from build123d import *

# Parameters (mm, degrees)
F1_DEPTH = 20
F2_W     = 20
F2_H     = 30
F3_DEPTH = 20
F5_DEPTH = 10
F6_DEPTH = 40
F7_R     = 10
F8_DEPTH = 30.001
F9_DEPTH = 10.001


with BuildPart() as f1:
    # F0 (on Right) → F1 (new body)
    with BuildSketch(Plane.YZ):
        Polygon((-13.2142865657, 0), (26.7857134343, 0), (26.7857134343, 30), (16.7857134343, 40), (-3.2142865657, 40), (-13.2142865657, 30), align=None)
    extrude(amount=-F1_DEPTH)

    # F2 (on face) → F3 (join)
    with BuildSketch(Plane.YZ):
        with Locations((6.7857134343, 15)):
            Rectangle(F2_W, F2_H)
    extrude(amount=F3_DEPTH)

    # F4 (on face) → F5 (join)
    with BuildSketch(Plane.XZ.offset(3.2142865657)):
        with BuildLine():
            ThreePointArc((35, 15), (30.6066017178, 25.6066017178), (20, 30))
            ThreePointArc((20, 30), (5, 15), (20, 0))
            ThreePointArc((20, 0), (30.6066017178, 4.3933982822), (35, 15))
        make_face()
    extrude(amount=F5_DEPTH)

    # F6 (add): a face of the model
    f6_faces = [f1.faces().sort_by_distance(p)[0] for p in [
        (20, -13.2142865657, 15),
    ]]
    extrude(f6_faces, amount=-F6_DEPTH)

    # F7 (on face) → F8 (cut, through all)
    with BuildSketch(Plane.XZ.offset(3.2142865657)):
        with Locations((20, 15)):
            Circle(F7_R)
    extrude(amount=-F8_DEPTH, mode=Mode.SUBTRACT)

    # F7 (on face) → F9 (cut, through all)
    with BuildSketch(Plane.XZ.offset(3.2142865657)):
        with Locations((20, 15)):
            Circle(F7_R)
    extrude(amount=F9_DEPTH, mode=Mode.SUBTRACT)


solid = f1.part
Can you work these out from the model? Positions are in its coordinate system, mm. A direction names the side the tool comes from. Give positions to 0.01 mm unless a question says otherwise; leave off trailing zeros. Loops run counter-clockwise (first coordinate to the right, second up) from the corner with the lowest first, then second, coordinate; pieces in that order, holes last. Notation, with made-up numbers: M 48.5,25.5 L 91.5,25.5 A25 ccw 91.5,48.5 Z; hole C -35,8 d11. An arc over 180 degrees is marked long. One line per item, written item: value. Start each with the question number.
1) Thinking about a two-plate mould opening in X: for faces 5 (the face through (3, -3.214, 15)), 6 (the face through (-10, -13.214, 15)), 7 (the face through (-20, 7, 20)), which applies, +X half, -X half, draft (parallel to the pull), parting line (faces both ways), or undercut?
2) I'm going to push flat-ended pins straight in: pin 1 (2 mm diameter, centred on y = 1.5, z = 7.5, fed in from +X); pin 2 (4 mm diameter, centred on x = 29.5, y = 15, fed in from +Z). Where does each tip first touch, or does it pass through?
3) If we section it at C-C, the plane y = 2.5: Write out the boundary of the cut face in (x, z).
4) If we section it at B-B, the plane z = 3: Write out the boundary of the cut face in (x, y).
5) If I drill on line 1 (X direction, y = -6.75, z = 15); line 2 (Z direction, x = 20, y = -9.25); line 3 (X direction, y = -7, z = 6.5), over which ranges is the centre line in solid material (lowest first)? Write a range as [from, to].
6) If we section it at A-A, the plane z = 15: Write out the boundary of the cut face in (x, y).
7) On a 3-axis mill with a long thin cutter (end or side, diameter ignored), from which of +Z, -Z, +X, -X, +Y, -Y can I reach the whole of each face in a straight line? I mean faces 1 (the face through (0, 7, 34)), 2 (the face through (3, 16.786, 15)), 3 (the face through (-9.86, -8.144, 35.07)), 4 (the face through (10, 7, 30)). Say none if no direction works.
Completed:
1. face 5: undercut
1. face 6: draft
1. face 7: -X half
2. pin 1: stops at x = 33.52
2. pin 2: stops at z = 27.99
3. outline: M -20,0 L 20,0 A15 ccw 20,30 L 0,30 L 0,40 L -20,40 Z; hole C 20,15 d20
4. outline: M -20,-13.21 L 0,-13.21 L 0,-3.21 L 11,-3.21 L 11,-13.21 L 29,-13.21 L 29,26.79 L 11,26.79 L 11,16.79 L 0,16.79 L 0,26.79 L -20,26.79 Z
5. line 1: x = [-20, 0], [5, 10], [30, 35]
5. line 2: z = [0, 5], [25, 30]
5. line 3: x = [-20, 0], [7.64, 14.73], [25.27, 32.36]
6. outline: M -20,-13.21 L 0,-13.21 L 0,-3.21 L 5,-3.21 L 5,-13.21 L 10,-13.21 L 10,26.79 L 5,26.79 L 5,16.79 L 0,16.79 L 0,26.79 L -20,26.79 Z; M 30,-13.21 L 35,-13.21 L 35,26.79 L 30,26.79 Z
7. face 1: +Z
7. face 2: +Y
7. face 3: +Z, +X, -X, -Y
7. face 4: +Z, +X, +Y, -Y
